Autodesk Inventor part; units mm, degrees
ref_plane "YZ Plane" through (0, 0, 0) normal (1, 0, 0) x (0, 1, 0)
ref_plane "XZ Plane" through (0, 0, 0) normal (0, 1, 0) x (-1, 0, 0)
ref_plane "XY Plane" through (0, 0, 0) normal (0, 0, 1) x (1, 0, 0)
sketch "Sketch1" plane through (0, 0, 0) normal (1, 0, 0) x (0, 1, 0)
  line L0 (3, -1.7321) -> (0, -3.4641)
  line L1 (0, -3.4641) -> (-3, -1.7321)
  line L2 (-3, -1.7321) -> (-3, 1.7321)
  line L3 (-3, 1.7321) -> (0, 3.4641)
  line L4 (0, 3.4641) -> (3, 1.7321)
  line L5 (3, 1.7321) -> (3, -1.7321)
  point P0 (0, 0)
  point P1 (0, 0)
  dimension "d0" = 6
extrude "Extrusion1" add sketch "Sketch1" along normal blind 7
sketch "Sketch2" plane through (7, 0, 0) normal (1, 0, 0) x (0, 0, -1)
  line L0 (-0.8, 5) -> (0.8, 5)
  line L1 (0.8, 5) -> (0.8, -5)
  line L2 (0.8, -5) -> (-0.8, -5)
  line L3 (-0.8, -5) -> (-0.8, 5)
  line L4 (-0.8, 5) -> (0.8, -5) construction
  line L5 (0.8, 5) -> (-0.8, -5) construction
  point P0 (0, 0)
  dimension "d3" = 1.6
  dimension "d4" = 10
extrude "Extrusion2" cut sketch "Sketch2" against normal blind 6
sketch "Sketch3" plane through (0, 0, 0) normal (-1, 0, 0) x (0, 0, 1)
  circle A0 centre (0, 0) radius 1.5
  dimension "d7" = 3
extrude "Extrusion3" add sketch "Sketch3" along normal blind 15
thread "Thread1"
sketch "Sketch4" plane through (7, -3, 0.8) normal (0, 0, -1) x (-1, 0, 0)
  line L0 (0, 6) -> (6, 6)
  line L1 (0, 0) -> (0, 6)
  line L2 (6, 0) -> (0, 0)
  line L3 (6, 0) -> (6, 6)
  line L4 (0, 0) -> (0, 6)
  circle A0 centre (3, 3) radius 1.5
  point P0 (7, 3)
  point P1 (3, 6)
  point P2 (0, 3)
  dimension "d12" = 3
extrude "Extrusion4" cut sketch "Sketch4" along normal through all both and the other way through all contours A0
properties part number "CompressionRollerArmActuatorScrew" material "Steel, Alloy"
The model under review builds one solid part; all positions refer to its coordinate system, in mm. A direction names the side the tool comes from. Round coordinates to 2 decimals unless told otherwise and drop trailing zeros. Order: outer loops, then holes, each group sorted by start corner. A loop starts at its lowest first (then second) coordinate and runs counter-clockwise, first axis right, second up. Notation, with made-up numbers: M 61,-2 L 110,-2 A20 ccw 110,17 Z; hole C -9.75,61.5 d2. An arc over 180 degrees is marked long. Use a Markdown table: item, result.
1) Wall thickness on line 1 along X through (y, z) = (0, -2.4); line 2 along Y through (x, z) = (4, 1.7); line 3 along X through (y, z) = (-2.15, -0.25): over which ranges is each line inside the solid? List them lowest first. Write a range as [from, to].
Report:
| item | result |
|---|---|
| line 1 | [0, 2.5], [5.5, 7] |
| line 2 | [-3, -1.5], [1.5, 3] |
| line 3 | [0, 1] |
2) Consider section A-A (x = 4). Write out the cut boundary in (y, z).
Report:
| item | result |
|---|---|
| outline | M -3,-1.73 L -1.5,-2.6 L -1.5,-0.8 L -3,-0.8 Z; M -3,0.8 L -1.5,0.8 L -1.5,2.6 L -3,1.73 Z; M 1.5,-2.6 L 3,-1.73 L 3,-0.8 L 1.5,-0.8 Z; M 1.5,0.8 L 3,0.8 L 3,1.73 L 1.5,2.6 Z |
3) Consider section D-D (z = 2.25). Write out the cut boundary in (x, y).
Report:
| item | result |
|---|---|
| outline | M 0,-2.1 L 7,-2.1 L 7,2.1 L 0,2.1 Z; hole C 4,0 d3 |
4) Draft analysis for pull direction Z (two halves, no side actions). For faces 4 (the face through (1, 0, 0)), 5 (the face through (3.45, 1.81, 2.42)), 6 (the face through (3.451, 1.854, -2.394)), state which applies: released by +Z, released by -Z, zero draft, split by the parting line, or undercut.
Report:
| item | result |
|---|---|
| face 4 | undercut |
| face 5 | released by +Z |
| face 6 | released by -Z |
5) Insertion check: pin 1 (1.8 mm diameter, centred on x = 4.5, y = 1.5, fed in from +Z); pin 2 (2 mm diameter, centred on x = -6, z = 2, fed in from -Y); pin 3 (1.8 mm diameter, centred on x = 4, y = 0, fed in from -Z); pin 4 (3 mm diameter, centred on x = -9.5, z = 0, fed in from -Y). Each pin has a flat end and moves straight along its axis. Give the tip position at first contact, or say it passes through.
Report:
| item | result |
|---|---|
| pin 1 | z = 2.93 |
| pin 2 | y = -1.12 |
| pin 3 | through |
| pin 4 | y = -1.5 |
6) Consider section C-C (y = -0.9). Write out the cut boundary in (x, z), then the cut area to 3 significant figures.
Report:
| item | result |
|---|---|
| outline | M -15,-1.2 L 0,-1.2 L 0,-2.94 L 2.8,-2.94 L 2.8,-0.8 L 1,-0.8 L 1,0.8 L 2.8,0.8 L 2.8,2.94 L 0,2.94 L 0,1.2 L -15,1.2 Z; M 5.2,-2.94 L 7,-2.94 L 7,-0.8 L 5.2,-0.8 Z; M 5.2,0.8 L 7,0.8 L 7,2.94 L 5.2,2.94 Z |
| area | 57.3 mm^2 |
7) Consider section B-B (z = 0). Write out the cut boundary in (x, y).
Report:
| item | result |
|---|---|
| outline | M -15,-1.5 L 0,-1.5 L 0,-3 L 1,-3 L 1,3 L 0,3 L 0,1.5 L -15,1.5 Z |
8) Tool access review of faces 1 (the face through (-7.4, -0.07, -1.5)), 2 (the face through (4.195, -1.487, -1.817)), 3 (the face through (5.4, -1.4, 0.8)): name each direction out of +Z, -Z, +X, -X, +Y, -Y from which nothing blocks a thin tool from reaching the whole face with its end or side.
Report:
| item | result |
|---|---|
| face 1 | -X |
| face 2 | +Z, -Z |
| face 3 | +X, +Y, -Y |
